from build123d import *

# Parameters (mm, degrees)
CUT_EXTRUDE1_DEPTH = 2.4
CHAMFER1_SIZE      = 0.5
FILLET1_R          = 0.5
CHAMFER2_SIZE      = 0.5


with BuildPart() as part:
    # Sketch1 → Revolve1 (revolve)
    with BuildSketch(Plane.XY, mode=Mode.PRIVATE) as revolve1_sk:
        Polygon((0, 0), (8, 0), (8, -7), (4.75, -7), (4.75, -7.5), (5, -7.5), (5, -77), (4, -77), (4, -90), (0, -90), align=None)
    revolve(revolve1_sk.sketch.rotate(Axis((0, 5, 0), (0, -1, 0)), 180), axis=Axis((0, 5, 0), (0, -1, 0)))

    # Sketch2 → Cut-Extrude1 (cut)
    with BuildSketch(Plane(origin=(0, 0, 0), x_dir=(1, 0, 0), z_dir=(0, 1, 0))):
        Polygon((0, -2.886751346), (2.5, -1.443375673), (2.5, 1.443375673), (0, 2.886751346), (-2.5, 1.443375673), (-2.5, -1.443375673), align=None)
    extrude(amount=-CUT_EXTRUDE1_DEPTH, mode=Mode.SUBTRACT)

    # Chamfer1
    chamfer1_edges = [part.edges().sort_by_distance(p)[0] for p in [
        (8, 0, 0),
    ]]
    chamfer(chamfer1_edges, length=CHAMFER1_SIZE)

    # Fillet1
    fillet1_edges = [part.edges().sort_by_distance(p)[0] for p in [
        (8, -7, 0),
    ]]
    fillet(fillet1_edges, radius=FILLET1_R)

    # Chamfer2
    chamfer2_edges = [part.edges().sort_by_distance(p)[0] for p in [
        (4, -90, 0),
    ]]
    chamfer(chamfer2_edges, length=CHAMFER2_SIZE)


solid = part.part
Geometry check sheet. Reference: the model listing, model coordinates, mm. A direction names the side the tool comes from. Round coordinates to 2 decimals unless told otherwise and drop trailing zeros. Order: outer loops, then holes, each group sorted by start corner. A loop starts at its lowest first (then second) coordinate and runs counter-clockwise, first axis right, second up. Notation, with made-up numbers: (19.25, 28.5) - (61.25, 28.5) arc R19 cw to (61.25, 41.5) - close; hole circle Ø10 at (50.5, 80). An arc over 180 degrees is marked (long way). One line per question, with ' | ' between items. Start each with the question number.
(1) Sectioned sample at A-A on z = 0. Record the cut outline in (x, y), and give its area (3 significant figures).
(2) Release check for a two-part mould opening along Z. For faces 5 (the cylindrical face through (1.73, -3.54, 7.81)), 6 (the flat face through (-1.233, -1.183, -2.175)), 7 (the flat face through (0, -7, 5)) record: released by +Z, released by -Z, zero draft, split by the parting line, or undercut.
(3) Sectioned sample at B-B on y = -10. Record the cut outline in (x, z).
(4) Depth check by flat-ended pin: pin 1 Ø6 at (y, z) = (-62.5, -3.5) entering from -X; pin 2 Ø1 at (x, z) = (1.5, 1) entering from +Y; pin 3 Ø1 at (x, z) = (4, 5) entering from -Y. Enter the tip coordinate at first touch or a pass-through.
(5) Access from +Z, -Z, +X, -X, +Y, -Y to the whole of each face (thin tool, end or side, straight path). Record for faces 1 (the cylindrical face through (5, -43, 0)), 2 (the flat face through (3, 0, 0)), 3 (the flat face through (1.233, -1.183, 2.175)), 4 (the cylindrical face through (1.03, -7.254, 4.637)).
(6) Thickness scan on L1, parallel to Y at x = -4.75, z = -5; L2, parallel to Y at x = -2, z = 1.5; L3, parallel to X at y = -76, z = -2. Record the ranges inside material, lowest first. Write a range as [from, to].
Conclusion:
1) outline: (-8, -6.5) arc R0.5 ccw to (-7.5, -7) - (-4.75, -7) - (-4.75, -7.5) - (-5, -7.5) - (-5, -77) - (-4, -77) - (-4, -89.5) - (-3.5, -90) - (3.5, -90) - (4, -89.5) - (4, -77) - (5, -77) - (5, -7.5) - (4.75, -7.5) - (4.75, -7) - (7.5, -7) arc R0.5 ccw to (8, -6.5) - (8, -0.5) - (7.5, 0) - (2.5, 0) - (2.5, -2.4) - (-2.5, -2.4) - (-2.5, 0) - (-7.5, 0) - (-8, -0.5) - close | area: 903 mm2
2) face 5: split by the parting line | face 6: undercut | face 7: zero draft
3) outline: circle Ø10 at (0, 0)
4) pin 1: stops at x = -4.97 | pin 2: stops at y = -2.4 | pin 3: stops at y = -7
5) face 1: -Y | face 2: +Z, -Z, +X, -X, +Y | face 3: +Y | face 4: none
6) L1: y = [-7, 0] | L2: y = [-90, -2.4] | L3: x = [-4.58, 4.58]
